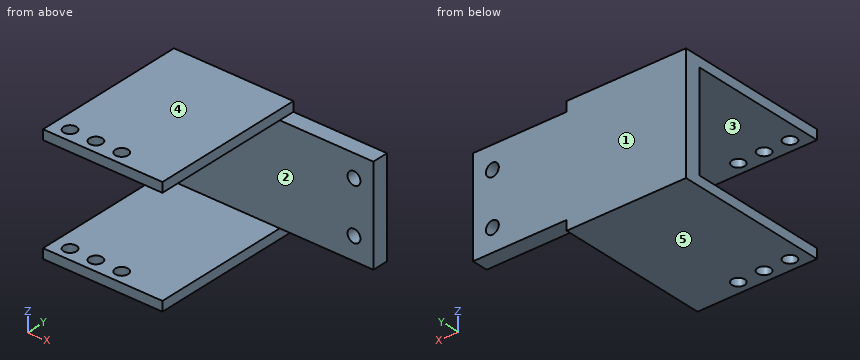
```python
from build123d import *

# Parameters (mm, degrees)
SKETCH_1_W          = 66
SKETCH_1_H          = 30
SKETCH_1_R          = 2
EXTRUDE_1_DEPTH     = 5
SKETCH_2_W          = 37
SKETCH_2_H          = 3
EXTRUDE_2_DEPTH     = 48
SKETCH_3_R          = 2
CUT_EXTRUDE_2_DEPTH = 44


with BuildPart() as part:
    # 草圖1 → 填料-伸長1 (new body)
    with BuildSketch(Plane(origin=(0, 0, 0), x_dir=(1, 0, 0), z_dir=(0, 1, 0))):
        with Locations((33, 15)):
            Rectangle(SKETCH_1_W, SKETCH_1_H)
        with Locations(Location((60, 23, 0), (0, 0, 270))):
            Circle(SKETCH_1_R, mode=Mode.SUBTRACT)
        with Locations(Location((60, 7, 0), (0, 0, 270))):
            Circle(SKETCH_1_R, mode=Mode.SUBTRACT)
    extrude(amount=EXTRUDE_1_DEPTH)

    # 草圖2 → 填料-伸長2 (add)
    with BuildSketch(Plane(origin=(0, 5, 0), x_dir=(1, 0, 0), z_dir=(0, 1, 0))):
        with Locations((18.5, 31.5)):
            Rectangle(SKETCH_2_W, SKETCH_2_H)
        with Locations((18.5, -1.5)):
            Rectangle(SKETCH_2_W, SKETCH_2_H)
    extrude(amount=-EXTRUDE_2_DEPTH)

    # 草圖3 → 除料-伸長2 (cut)
    with BuildSketch(Plane.XY.offset(3)):
        with Locations((21, -39)):
            Circle(SKETCH_3_R)
        with Locations((13, -39)):
            Circle(SKETCH_3_R)
        with Locations((5, -39)):
            Circle(SKETCH_3_R)
    extrude(amount=-CUT_EXTRUDE_2_DEPTH, mode=Mode.SUBTRACT)


solid = part.part
```
Geometry check sheet. Reference: the model listing, model coordinates, mm. Face numbers are marked on the shaded views. A direction names the side the tool comes from. Coordinates: 2 decimals unless noted, no trailing zeros. Order: outer loops, then holes, each group sorted by start corner. A loop starts at its lowest first (then second) coordinate and runs counter-clockwise, first axis right, second up. Notation, with made-up numbers: M -11.75,-24.5 L 22.25,-24.5 A26 cw 22.25,9.5 Z; hole C -7.75,-16.5 d8. An arc over 180 degrees is marked long. Answer as a JSON object with one key per item and string values.
Q1. Depth check by flat-ended pin: pin 1 Ø3.5 at (x, y) = (5, -39) entering from -Z; pin 2 Ø2 at (x, z) = (20, -11.5) entering from -Y; pin 3 Ø4 at (x, y) = (56, 2.5) entering from +Z; pin 4 Ø2.5 at (x, y) = (47, 3.5) entering from -Z. Enter the tip coordinate at first touch or a pass-through.
Results are:
{"pin 1": "passes through", "pin 2": "stops at y = 0", "pin 3": "stops at z = 0", "pin 4": "stops at z = -30"}
Q2. Cross-section at C-C on z = -23. Record the cut outline in (x, y).
Results are:
{"outline": "M 0,0 L 58,0 L 58,5 L 0,5 Z; M 62,0 L 66,0 L 66,5 L 62,5 Z"}
Q3. Cross-section at B-B on x = 21. Record the cut outline in (y, z).
Results are:
{"outline": "M -43,-33 L -41,-33 L -41,-30 L -43,-30 Z; M -43,0 L -41,0 L -41,3 L -43,3 Z; M -37,-33 L 5,-33 L 5,3 L -37,3 L -37,0 L 0,0 L 0,-30 L -37,-30 Z"}
Q4. Scan lines: line 1 (Y direction, x = 21, z = 1); line 2 (X direction, y = 1.7, z = -23); line 3 (Z direction, x = 22, y = -18). Record each from-to range of solid material in increasing order.
Results are:
{"line 1": "y = -43 to -41, -37 to 5", "line 2": "x = 0 to 58, 62 to 66", "line 3": "z = -33 to -30, 0 to 3"}
Q5. Release check for a two-part mould opening along Z. For the marked faces 3, 4 and 5 record: released by +Z, released by -Z, zero draft, split by the parting line, or undercut.
Results are:
{"face 3": "undercut", "face 4": "released by +Z", "face 5": "released by -Z"}
Q6. Cross-section at A-A on y = -4. Record the cut outline in (x, z).
Results are:
{"outline": "M 0,-33 L 37,-33 L 37,-30 L 0,-30 Z; M 0,0 L 37,0 L 37,3 L 0,3 Z"}
Q7. Cross-section at D-D on y = 1.5. Record the cut outline in (x, z).
Results are:
{"outline": "M 0,-33 L 37,-33 L 37,-30 L 66,-30 L 66,0 L 37,0 L 37,3 L 0,3 Z; hole C 60,-23 d4; hole C 60,-7 d4"}
Q8. Tool access check on the marked faces 1 and 2. Record the directions out of +Z, -Z, +X, -X, +Y, -Y that give a thin tool (end or side, any length) a straight path to the whole face; none if there is none.
Results are:
{"face 1": "+Z, -Z, +X, -X, +Y", "face 2": "+X, -X, -Y"}
